from build123d import *

# Parameters (mm, degrees)
SKETCH1_R           = 3
BOSS_EXTRUDE1_DEPTH = 6
SCALE1_SCALE        = 0.5


with BuildPart() as part:
    # Sketch1 → Boss-Extrude1 (new body)
    with BuildSketch(Plane.XY):
        with BuildLine():
            Line((-180, 8.791952491), (180, 8.791952491))
            ThreePointArc((180, 8.791952491), (188.791952491, 0), (180, -8.791952491))
            Line((180, -8.791952491), (-65.874044075, -12.652154123))
            ThreePointArc((-65.874044075, -12.652154123), (-79.997495837, -12.674394151), (-94.115941273, -12.297720824))
            Line((-94.115941273, -12.297720824), (-180, -8.791952491))
            ThreePointArc((-180, -8.791952491), (-188.791952491, 0), (-180, 8.791952491))
        make_face()
        with Locations((-180, 0)):
            Circle(SKETCH1_R, mode=Mode.SUBTRACT)
        with Locations((-80, 0)):
            Circle(SKETCH1_R, mode=Mode.SUBTRACT)
        with Locations((180, 0)):
            Circle(SKETCH1_R, mode=Mode.SUBTRACT)
    extrude(amount=-BOSS_EXTRUDE1_DEPTH)


with BuildPart() as part_1:
    # Scale1: scaled about (-2.379309964, -1.029732749, -3)
    add(part.part.scale(SCALE1_SCALE).moved(Location((-1.189654982, -0.514866374, -1.5))))


solid = part_1.part
Work out the finished part from the listing and answer in its coordinate system (mm). Give positions to 0.01 mm unless a question says otherwise; leave off trailing zeros. Loops run counter-clockwise (first coordinate to the right, second up) from the corner with the lowest first, then second, coordinate; pieces in that order, holes last. Notation, with made-up numbers: (51, 51.5) - (101, 51.5) arc R20 ccw to (101, 62.5) - close; hole circle Ø3 at (46, -2.75). An arc over 180 degrees is marked (long way). Answer in a Markdown table with one row per item. Add a question column.
Q1. Consider line 1 along Y through (x, z) = (86.5, -2.4); line 2 along Y through (x, z) = (54.5, -3.3); line 3 along X through (y, z) = (-2.75, -4.15) (3 decimals). Determine where each line is inside the solid, lowest interval first.
Q2. Determine the mould class of faces 1 (the cylindrical face through (93.205, -0.418, -2.979)), 2 (the flat face through (-2, 3.881, -3)), 3 (the cylindrical face through (87.31, -0.45, -2.98)) for opening direction X: released by +X, released by -X, zero draft, split by the parting line, or undercut.
Q3. The part is cut by section A-A (z = -3.2). Determine the outline of the cut face in (x, y), and give its area (3 significant figures).
Q4. The part is cut by section B-B (x = 79). Determine the outline of the cut face in (y, z), and give its area (3 significant figures).
Q5. The part is cut by section C-C (x = 45.5). Determine the outline of the cut face in (y, z).
Q6. This flat-tipped pin is pushed along its axis until it touches: P1, Ø1, axis at x = -4.5, z = -4, coming from the -Y side. Where does it stop, or does it pass through?
Solution:
| question | item | result |
|---|---|---|
| 1 | line 1 | y = -4.95 to 3.88 |
| 1 | line 2 | y = -5.45 to 3.88 |
| 1 | line 3 | x = -94.975 to 92.596 |
| 2 | face 1 | released by +X |
| 2 | face 2 | zero draft |
| 2 | face 3 | undercut |
| 3 | outline | (-91.19, -4.91) - (-48.25, -6.66) arc R250 ccw to (-34.13, -6.84) - (88.81, -4.91) arc R4.4 ccw to (88.81, 3.88) - (-91.19, 3.88) arc R4.4 ccw to start; hole circle Ø3 at (-91.19, -0.51); hole circle Ø3 at (-41.19, -0.51); hole circle Ø3 at (88.81, -0.51) |
| 3 | area | 1,810 mm² |
| 4 | outline | (-5.06, -4.5) - (3.88, -4.5) - (3.88, -1.5) - (-5.06, -1.5) - close |
| 4 | area | 26.8 mm² |
| 5 | outline | (-5.59, -4.5) - (3.88, -4.5) - (3.88, -1.5) - (-5.59, -1.5) - close |
| 6 | P1 | stops at y = -6.38 |
